from build123d import *

# Parameters (mm, degrees)
SKETCH1_W           = 215.9
SKETCH1_H           = 215.9
BOSS_EXTRUDE1_DEPTH = 12.7
BOSS_EXTRUDE2_DEPTH = 38.1
SKETCH4_W           = 47.244
SKETCH4_H           = 41.06164
CUT_EXTRUDE1_DEPTH  = 8.89
SKETCH6_W           = 47.244
SKETCH6_H           = 6.35
BOSS_EXTRUDE3_DEPTH = 38.1
SKETCH5_R           = 10.922
CUT_EXTRUDE2_DEPTH  = 175.83836
CUT_EXTRUDE4_DEPTH  = 38.1
SKETCH9_W           = 47.244
SKETCH9_H           = 85.1916
CUT_EXTRUDE5_DEPTH  = 6.35
SKETCH12_R          = 38.1
BOSS_EXTRUDE4_DEPTH = 12.7
SKETCH14_W          = 38.1
SKETCH14_H          = 6.35
CUT_EXTRUDE7_DEPTH  = 6.35
SKETCH10_R          = 1.905
CUT_EXTRUDE9_DEPTH  = 12.7
CUT_EXTRUDE10_DEPTH = 6.35


with BuildPart() as part:
    # Sketch1 → Boss-Extrude1 (new body)
    with BuildSketch(Plane.XY):
        with Locations((107.95, 107.95)):
            Rectangle(SKETCH1_W, SKETCH1_H)
    extrude(amount=BOSS_EXTRUDE1_DEPTH)

    # Sketch2 → Boss-Extrude2 (add)
    with BuildSketch(Plane.XY.offset(12.7)):
        Polygon((174.2694, 41.06164), (197.8914, 41.06164), (197.8914, 53.76164), (150.6474, 53.76164), (150.6474, 41.06164), align=None)
    extrude(amount=BOSS_EXTRUDE2_DEPTH)

    # Sketch4 → Cut-Extrude1 (cut)
    with BuildSketch(Plane.XY.offset(12.7)):
        with Locations((174.2694, 20.53082)):
            Rectangle(SKETCH4_W, SKETCH4_H)
    extrude(amount=-CUT_EXTRUDE1_DEPTH, mode=Mode.SUBTRACT)

    # Sketch6 → Boss-Extrude3 (add)
    with BuildSketch(Plane.XY.offset(12.7)):
        with Locations((174.2694, 142.12824)):
            Rectangle(SKETCH6_W, SKETCH6_H)
    extrude(amount=BOSS_EXTRUDE3_DEPTH)

    # Sketch5 → Cut-Extrude2 (cut, through all)
    with BuildSketch(Plane.XZ.offset(-41.06164)):
        with Locations((171.730776396, 25.411523701)):
            Circle(SKETCH5_R)
    extrude(amount=-CUT_EXTRUDE2_DEPTH, mode=Mode.SUBTRACT)

    # Sketch8 → Cut-Extrude4 (cut)
    with BuildSketch(Plane.XZ.offset(-41.06164)):
        with BuildLine():
            Line((160.812004434, 25.146), (160.812004434, 50.8))
            Line((160.812004434, 50.8), (182.649548358, 50.8))
            Line((182.649548358, 50.8), (182.649548358, 25.146))
            ThreePointArc((182.649548358, 25.146), (171.730776396, 36.064771962), (160.812004434, 25.146))
        make_face()
    extrude(amount=-CUT_EXTRUDE4_DEPTH, mode=Mode.SUBTRACT)

    # Sketch9 → Cut-Extrude5 (cut)
    with BuildSketch(Plane.XY.offset(12.7)):
        with Locations((174.2694, 96.35744)):
            Rectangle(SKETCH9_W, SKETCH9_H)
    extrude(amount=-CUT_EXTRUDE5_DEPTH, mode=Mode.SUBTRACT)

    # Sketch12 → Boss-Extrude4 (add)
    with BuildSketch(Plane.XY.offset(12.7)):
        with Locations((107.95, 105.927514247)):
            Circle(SKETCH12_R)
    extrude(amount=BOSS_EXTRUDE4_DEPTH)

    # Sketch14 → Cut-Extrude7 (cut)
    with BuildSketch(Plane.ZY.offset(-150.6474)):
        with Locations((31.75, 142.12824)):
            Rectangle(SKETCH14_W, SKETCH14_H)
    extrude(amount=-CUT_EXTRUDE7_DEPTH, mode=Mode.SUBTRACT)

    # Sketch10 → Cut-Extrude9 (cut)
    with BuildSketch(Plane.XZ.offset(-41.06164)):
        with Locations((187.059676396, 9.498423701)):
            Circle(SKETCH10_R)
        with Locations((156.401876396, 9.498423701)):
            Circle(SKETCH10_R)
        with Locations((156.401876396, 40.156223701)):
            Circle(SKETCH10_R)
        with Locations((187.059676396, 40.156223701)):
            Circle(SKETCH10_R)
    extrude(amount=-CUT_EXTRUDE9_DEPTH, mode=Mode.SUBTRACT)

    # Sketch15 → Cut-Extrude10 (cut)
    with BuildSketch(Plane.XY.offset(12.7)):
        with BuildLine():
            Line((197.8914, 145.30324), (197.8914, 0))
            Line((197.8914, 0), (215.9, 0))
            Line((215.9, 0), (215.9, 215.9))
            Line((215.9, 215.9), (0, 215.9))
            Line((0, 215.9), (0, 0))
            Line((0, 0), (150.6474, 0))
            Line((150.6474, 0), (150.6474, 78.403487774))
            ThreePointArc((150.6474, 78.403487774), (57.15, 105.927514247), (150.6474, 133.451540719))
            Line((150.6474, 133.451540719), (150.6474, 138.95324))
            Line((150.6474, 138.95324), (156.9974, 145.30324))
            Line((156.9974, 145.30324), (197.8914, 145.30324))
        make_face()
    extrude(amount=-CUT_EXTRUDE10_DEPTH, mode=Mode.SUBTRACT)


solid = part.part
Geometry: final body of the model. Coordinates: model frame, mm. A direction names the side the tool comes from. Give positions to 0.01 mm unless a question says otherwise; leave off trailing zeros. Order: outer loops, then holes, each group sorted by start corner. A loop starts at its lowest first (then second) coordinate and runs counter-clockwise, first axis right, second up. Notation, with made-up numbers: (-17, 87.5) -> (24, 87.5) arc R23 ccw to (24, 110.5) -> close; hole circle Ø2 at (52, 18.25). An arc over 180 degrees is marked (long way). Write each question's results on one line, items separated by ' | '.
1) Set-up query: faces 4 (the face through (185, 53.762, 23)), 5 (the face through (153.778, 142.084, 9.569)), 6 (the face through (182, 145.303, 34)). Return all of +Z, -Z, +X, -X, +Y, -Y with unobstructed straight access to the full face (end or side cutting, diameter ignored); none if empty.
Geometry says:
face 4: +Z, +X, -X | face 5: +Z, +Y | face 6: +Z, +X, +Y
2) Cut plane A-A (x = 107.95). Output: boundary loops of the cut face in (y, z).
Geometry says:
outline: (0, 0) -> (215.9, 0) -> (215.9, 6.35) -> (156.73, 6.35) -> (156.73, 12.7) -> (144.03, 12.7) -> (144.03, 25.4) -> (67.83, 25.4) -> (67.83, 12.7) -> (55.13, 12.7) -> (55.13, 6.35) -> (0, 6.35) -> close
3) Cut plane B-B (y = 34). Output: boundary loops of the cut face in (x, z).
Geometry says:
outline: (0, 0) -> (215.9, 0) -> (215.9, 6.35) -> (197.89, 6.35) -> (197.89, 3.81) -> (150.65, 3.81) -> (150.65, 6.35) -> (0, 6.35) -> close
4) Cut plane D-D (y = 63.5). Output: boundary loops of the cut face in (x, z), and give its area (3 significant figures).
Geometry says:
outline: (0, 0) -> (215.9, 0) -> (215.9, 6.35) -> (135.89, 6.35) -> (135.89, 12.7) -> (80.01, 12.7) -> (80.01, 6.35) -> (0, 6.35) -> close | area: 1,730 mm²
5) Cut plane C-C (x = 170). Output: boundary loops of the cut face in (y, z).
Geometry says:
outline: (0, 0) -> (215.9, 0) -> (215.9, 6.35) -> (145.3, 6.35) -> (145.3, 14.63) -> (138.95, 14.63) -> (138.95, 6.35) -> (53.76, 6.35) -> (53.76, 14.63) -> (41.06, 14.63) -> (41.06, 3.81) -> (0, 3.81) -> close; (138.95, 36.2) -> (145.3, 36.2) -> (145.3, 50.8) -> (138.95, 50.8) -> close
6) Draft query along Z for faces 1 (the face through (174, 21, 3.81)), 2 (the face through (181.82, 142.08, 21.23)), 3 (the face through (150.647, 47, 29)). Return one class per face: released by +Z, released by -Z, zero draft, split by the parting line, or undercut.
Geometry says:
face 1: released by +Z | face 2: undercut | face 3: zero draft
7) First-contact query: pin 1 Ø1 at (x, y) = (187.5, 88) entering from +Z; pin 2 Ø10 at (y, z) = (49, 38) entering from -X; pin 3 Ø6 at (x, z) = (156.4, 40.16) entering from +Y; pin 4 Ø2 at (y, z) = (17, 4.5) entering from -X. Flat tips, straight axial feed; report the tip coordinate or a pass-through.
Geometry says:
pin 1: stops at z = 6.35 | pin 2: stops at x = 150.65 | pin 3: stops at y = 145.3 | pin 4: stops at x = 0
8) Line query: line 1 along Y through (x, z) = (195, 26.5); line 2 along Z through (x, y) = (77, 59.5); line 3 along X through (y, z) = (143.5, 27.5). Output: solid intervals per line, ascending.
Geometry says:
line 1: y = 41.06 to 53.76, 138.95 to 145.3 | line 2: z = 0 to 6.35 | line 3: x = 157 to 161.01, 182.45 to 197.89
